Here's how the part is built. I have some questions about the finished solid (model axes, mm). A direction names the side the tool comes from. Coordinates: 2 decimals unless noted, no trailing zeros. Write each loop counter-clockwise with the first axis right and the second up, starting at its lowest first coordinate (ties: lowest second). Pieces come first, ordered by that corner, then holes. Notation, with made-up numbers: (-21, 24) - (25, 24) arc R20 cw to (25, 59) - close; hole circle Ø11 at (-14.75, 28.25). An arc over 180 degrees is marked (long way). Answer in a Markdown table with one row per item. Add a question column.
Item 1: Imagine slicing it at C-C (y = -24). Please give me the cut outline in (x, z) (3 decimals).
Item 2: Imagine slicing it at A-A (z = -10). Please give me the cut outline in (x, y) (3 decimals).
Item 3: Imagine slicing it at B-B (x = -10). Please give me the cut outline in (y, z) (3 decimals), plus the area to 3 significant figures.
Item 4: If I drill on probe 1 along X at (y, z) = (-6.1, 10) (3 decimals); probe 2 along Z at (x, y) = (-3.5, -18.5) (3 decimals), over which ranges is the centre line in solid material (lowest first)? Write a range as from..to.
Item 5: I'm going to push flat-ended pins straight in: pin 1 (6 mm diameter, centred on x = -1.5, y = -15.5, fed in from -Z); pin 2 (4 mm diameter, centred on x = -11.5, z = 8.5, fed in from +Y); pin 3 (4 mm diameter, centred on x = 8.5, y = -33, fed in from -Z); pin 4 (13 mm diameter, centred on x = -1, y = -29.5, fed in from +Z). Where does each tip first touch, or does it pass through?
Item 6: Which directions (+Z, -Z, +X, -X, +Y, -Y) give clear straight access to the entire face, cutting with the end or side of a thin tool? Please do faces 5 (the face through (-3.75, -18, 0)), 6 (the face through (0, -2, 6)), 7 (the face through (0, -24, -6)), 8 (the face through (0, -24, 6)), 9 (the face through (6, -2, 0)).
Item 7: We'd pull the mould along X, two halves only. Please class faces 1 (the face through (15, -6, 0)), 2 (the face through (9.78, -5.83, 8.29)), 3 (the face through (8.73, -5.83, -11.17)), 4 (the face through (0, -4.35, 7)): +X half, -X half, draft (parallel to the pull), parting line (faces both ways), or undercut.
Item 8: Imagine slicing it at D-D (z = 7.5). Please give me the cut outline in (x, y).
from build123d import *

# Parameters (mm, degrees)
SKETCH_W        = 12
SKETCH_H        = 12
PAD_DEPTH       = 41
SKETCH001_W     = 7.5
SKETCH001_H     = 3.75
POCKET_DEPTH    = 36.1
SKETCH003_W     = 12
SKETCH003_H     = 3
PAD001_DEPTH    = 9
PAD001_FACE11_W = 3
PAD001_FACE11_H = 9
PAD002_DEPTH    = 9
PAD002_FACE11_W = 3
PAD002_FACE11_H = 9
PAD003_DEPTH    = 21
PAD003_FACE17_W = 3
PAD003_FACE17_H = 9
PAD004_DEPTH    = 21
PAD004_FACE12_W = 3
PAD004_FACE12_H = 9
PAD005_DEPTH    = 9
PAD005_FACE17_W = 3
PAD005_FACE17_H = 9
PAD006_DEPTH    = 12
SKETCH004_R     = 1.725
POCKET001_DEPTH = 36.651


with BuildPart() as part:
    # Sketch → Pad (new body)
    with BuildSketch(Plane.XZ):
        Rectangle(SKETCH_W, SKETCH_H)
    extrude(amount=PAD_DEPTH)

    # Sketch001 (on Face5 of Pad) → Pocket (cut)
    with BuildSketch(Plane(origin=(0, 0, 0), x_dir=(1, 0, 0), z_dir=(0, 1, 0))):
        Rectangle(SKETCH001_W, SKETCH001_H)
    extrude(amount=-POCKET_DEPTH, mode=Mode.SUBTRACT)

    # Sketch003 (on Face1 of Pocket) → Pad001 (join)
    with BuildSketch(Plane(origin=(0, 0, 6), x_dir=(-1, 0, 0), z_dir=(0, 0, 1))):
        with Locations((0, 5.85)):
            Rectangle(SKETCH003_W, SKETCH003_H)
    extrude(amount=PAD001_DEPTH)

    # Pad001 Face11 → Pad002 (add)
    with BuildSketch(Plane(origin=(6, -5.85, 10.5), x_dir=(0, -1, 0), z_dir=(1, 0, 0))):
        Rectangle(PAD001_FACE11_W, PAD001_FACE11_H)
    extrude(amount=PAD002_DEPTH)

    # Pad002 Face11 → Pad003 (add)
    with BuildSketch(Plane(origin=(10.5, -5.85, 6), x_dir=(0, -1, 0), z_dir=(0, 0, -1))):
        Rectangle(PAD002_FACE11_W, PAD002_FACE11_H)
    extrude(amount=PAD003_DEPTH)

    # Pad003 Face17 → Pad004 (add)
    with BuildSketch(Plane(origin=(6, -5.85, -10.5), x_dir=(0, 1, 0), z_dir=(-1, 0, 0))):
        Rectangle(PAD003_FACE17_W, PAD003_FACE17_H)
    extrude(amount=PAD004_DEPTH)

    # Pad004 Face12 → Pad005 (add)
    with BuildSketch(Plane(origin=(-6, -5.85, 10.5), x_dir=(0, 1, 0), z_dir=(-1, 0, 0))):
        Rectangle(PAD004_FACE12_W, PAD004_FACE12_H)
    extrude(amount=PAD005_DEPTH)

    # Pad005 Face17 → Pad006 (add)
    with BuildSketch(Plane(origin=(-10.5, -5.85, 6), x_dir=(0, -1, 0), z_dir=(0, 0, -1))):
        Rectangle(PAD005_FACE17_W, PAD005_FACE17_H)
    extrude(amount=PAD006_DEPTH)

    # Sketch004 (on Face13 of Pad006) → Pocket001 (cut, through all)
    with BuildSketch(Plane(origin=(0, -4.35, 0), x_dir=(1, 0, 0), z_dir=(0, 1, 0))):
        with Locations((-10, 10)):
            Circle(SKETCH004_R)
        with Locations((10, 10)):
            Circle(SKETCH004_R)
        with Locations((10, -10)):
            Circle(SKETCH004_R)
        with Locations((-10, -10)):
            Circle(SKETCH004_R)
    extrude(amount=-POCKET001_DEPTH, mode=Mode.SUBTRACT)


solid = part.part
Here are the results:
| question | item | result |
|---|---|---|
| 1 | outline | (-6, -6) - (6, -6) - (6, 6) - (-6, 6) - close; hole (-3.75, -1.875) - (3.75, -1.875) - (3.75, 1.875) - (-3.75, 1.875) - close |
| 2 | outline | (-15, -7.35) - (-11.725, -7.35) - (-11.725, -4.35) - (-15, -4.35) - close; (-8.275, -7.35) - (8.275, -7.35) - (8.275, -4.35) - (-8.275, -4.35) - close; (11.725, -7.35) - (15, -7.35) - (15, -4.35) - (11.725, -4.35) - close |
| 3 | outline | (-7.35, -15) - (-4.35, -15) - (-4.35, -11.725) - (-7.35, -11.725) - close; (-7.35, -8.275) - (-4.35, -8.275) - (-4.35, 8.275) - (-7.35, 8.275) - close; (-7.35, 11.725) - (-4.35, 11.725) - (-4.35, 15) - (-7.35, 15) - close |
| 3 | area | 69.3 mm2 |
| 4 | probe 1 | x = -15..-11.725, -8.275..8.275, 11.725..15 |
| 4 | probe 2 | z = -6..-1.875, 1.875..6 |
| 5 | pin 1 | stops at z = -6 |
| 5 | pin 2 | stops at y = -4.35 |
| 5 | pin 3 | passes through |
| 5 | pin 4 | stops at z = 6 |
| 6 | face 5 | +Y |
| 6 | face 6 | +Z, +X, -X, +Y |
| 6 | face 7 | -Z, +X, -X, -Y |
| 6 | face 8 | +Z, +X, -X, -Y |
| 6 | face 9 | +Z, -Z, +X, +Y |
| 7 | face 1 | +X half |
| 7 | face 2 | undercut |
| 7 | face 3 | undercut |
| 7 | face 4 | draft |
| 8 | outline | (-15, -7.35) - (15, -7.35) - (15, -4.35) - (-15, -4.35) - close |
